Part model, mm, in its own coordinate system. A direction names the side the tool comes from. Round coordinates to 2 decimals unless told otherwise and drop trailing zeros. Loops run counter-clockwise (first coordinate to the right, second up) from the corner with the lowest first, then second, coordinate; pieces in that order, holes last.
(1) Cut at B-B on x = 346.5. List the corners of the cut face in (y, z), then the cut area to 3 significant figures.
(2) Cut at A-A on y = 3.65. List the corners of the cut face in (x, z), then the cut area to 3 significant figures.
(3) Tool access for faces 1 (the face through (296, 5, -50)), 2 (the face through (296, 2, -15)): list every direction of +Z, -Z, +X, -X, +Y, -Y with a clear straight run to the whole face (end or side of a thin tool).
(4) Probe probe 1 along Z at (x, y) = (540, 0.4); probe 2 along Z at (x, y) = (239, 3.9); probe 3 along Y at (x, z) = (277, -84.5). List the from-to ranges inside material, lowest first.
(5) Flat gauge pins, fed straight in: pin 1 (2 mm diameter, centred on x = 216.5, z = -20, fed in from -Y); pin 2 (4.5 mm diameter, centred on x = 540, z = -15, fed in from +Y). Where does each tip first touch, or does it go through?
from build123d import *

# Parameters (mm, degrees)
SKETCH1_W           = 600
SKETCH1_H           = 5
BOSS_EXTRUDE1_DEPTH = 100
SKETCH5_W           = 600
SKETCH5_H           = 10
CUT_EXTRUDE1_DEPTH  = 3
SKETCH6_R           = 2
CUT_EXTRUDE2_DEPTH  = 609.296802556


with BuildPart() as part:
    # Sketch1 → Boss-Extrude1 (new body)
    with BuildSketch(Plane.XY):
        with Locations((300, 2.5)):
            Rectangle(SKETCH1_W, SKETCH1_H)
    extrude(amount=-BOSS_EXTRUDE1_DEPTH)

    # Sketch5 → Cut-Extrude1 (cut)
    with BuildSketch(Plane(origin=(0, 5, 0), x_dir=(1, 0, 0), z_dir=(0, 1, 0))):
        with Locations((300, 85)):
            Rectangle(SKETCH5_W, SKETCH5_H)
        with Locations((300, 15)):
            Rectangle(SKETCH5_W, SKETCH5_H)
    extrude(amount=-CUT_EXTRUDE1_DEPTH, mode=Mode.SUBTRACT)

    # Sketch6 → Cut-Extrude2 (cut, through all)
    with BuildSketch(Plane(origin=(0, 5, 0), x_dir=(1, 0, 0), z_dir=(0, 1, 0))):
        with Locations(Location((60, 85, 0), (0, 0, 180))):
            Circle(SKETCH6_R)
        with Locations(Location((60, 15, 0), (0, 0, 180))):
            Circle(SKETCH6_R)
        with Locations(Location((540, 85, 0), (0, 0, 180))):
            Circle(SKETCH6_R)
        with Locations(Location((540, 15, 0), (0, 0, 180))):
            Circle(SKETCH6_R)
    extrude(amount=-CUT_EXTRUDE2_DEPTH, mode=Mode.SUBTRACT)


solid = part.part
Final values:
1. outline: (0, -100) - (5, -100) - (5, -90) - (2, -90) - (2, -80) - (5, -80) - (5, -20) - (2, -20) - (2, -10) - (5, -10) - (5, 0) - (0, 0) - close
1. area: 440 mm2
2. outline: (0, -100) - (600, -100) - (600, -90) - (0, -90) - close; (0, -80) - (600, -80) - (600, -20) - (0, -20) - close; (0, -10) - (600, -10) - (600, 0) - (0, 0) - close
2. area: 48,000 mm2
3. face 1: +Z, -Z, +X, -X, +Y
3. face 2: +X, -X, +Y
4. probe 1: z = -100 to -87, -83 to -17, -13 to 0
4. probe 2: z = -100 to -90, -80 to -20, -10 to 0
4. probe 3: y = 0 to 2
5. pin 1: stops at y = 0
5. pin 2: stops at y = 2
